The figure shows three views and two pictorial views of one solid part (mm, origin at its lowest corner). Answer the questions. Coordinates: 2 decimals unless noted, no trailing zeros. Write each loop counter-clockwise with the first axis right and the second up, starting at its lowest first coordinate (ties: lowest second). Pieces come first, ordered by that corner, then holes.
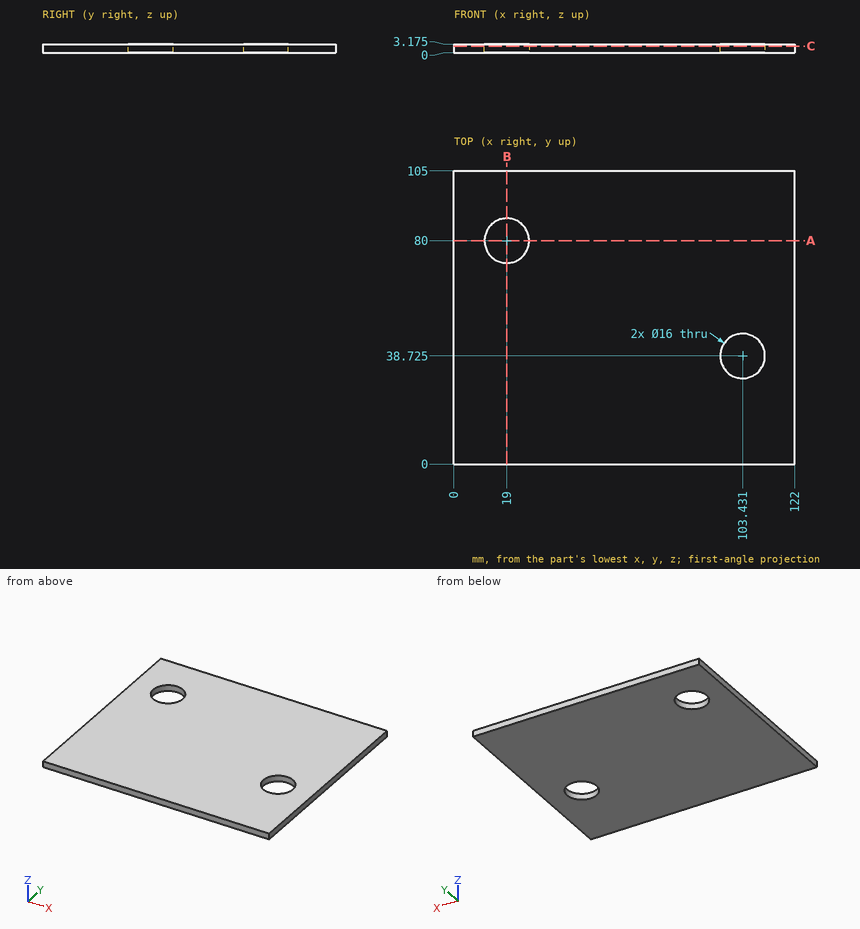
Q1. The part is cut by section A-A, the plane y = 80. Write down the section's boundary in (x, z) (3 decimals).
Answers below:
outline: (0, 0) - (11, 0) - (11, 3.175) - (0, 3.175) - close; (27, 0) - (122, 0) - (122, 3.175) - (27, 3.175) - close
Q2. The part is cut by section B-B, the plane x = 19. Write down the section's boundary in (y, z) (3 decimals).
Answers below:
outline: (0, 0) - (72, 0) - (72, 3.175) - (0, 3.175) - close; (88, 0) - (105, 0) - (105, 3.175) - (88, 3.175) - close
Q3. Find the intervals of material crossed by probe 1 along Y at (x, z) = (19, 0.7); probe 2 along X at (y, z) = (42.5, 0.4); probe 3 along X at (y, z) = (37, 1.7), in increasing order.
Answers below:
probe 1: y = 0 to 72, 88 to 105
probe 2: x = 0 to 96.38, 110.48 to 122
probe 3: x = 0 to 95.62, 111.24 to 122
Q4. Given pin 1 (21 mm diameter, centred on x = 103.43, y = 38.72, fed in from -Z); pin 2 (14.5 mm diameter, centred on x = 19, y = 80, fed in from -Z), each flat-ended and moving along its own axis, determine where each tip first touches the part or whether it passes through.
Answers below:
pin 1: stops at z = 0
pin 2: passes through
Q5. The part is cut by section C-C, the plane z = 2.45. Write down the section's boundary in (x, y) (3 decimals), then the cut area to 3 significant figures.
Answers below:
outline: (0, 0) - (122, 0) - (122, 105) - (0, 105) - close; hole circle Ø16 at (19, 80); hole circle Ø16 at (103.431, 38.725)
area: 12,400 mm2
